Read the model definition and answer for the solid it produces. Units are mm, in the model's axes. A direction names the side the tool comes from. Coordinates: 2 decimals unless noted, no trailing zeros. Loops run counter-clockwise (first coordinate to the right, second up) from the corner with the lowest first, then second, coordinate; pieces in that order, holes last. Notation, with made-up numbers: (47.5, 69) -> (56.5, 69) arc R19 cw to (56.5, 100) -> close; hole circle Ø1 at (-15.5, -22.5). An arc over 180 degrees is marked (long way). Answer as a JSON object with one key per item and string values. Group by question number.
1) Determine the mould class of faces 5 (the face through (3, -20, -24.284)), 6 (the face through (0, -20, -14)), 7 (the face through (2, -7, -7)) for opening direction Y: released by +Y, released by -Y, zero draft, split by the parting line, or undercut.
2) Section D-D, the plane y = -23 is taken. Give the vertices of the cut face in (x, z).
3) A flat-ended cylindrical pin translates along its axis: P1, Ø1.5, axis at x = 2.5, z = -9, coming from the +Y side. Find the tip coordinate at first contact, or state that the pin passes through.
4) Section B-B, the plane x = 4.1 is taken. Give the vertices of the cut face in (y, z).
5) Consider probe 1 along Z at (x, y) = (4.1, -18.5); probe 2 along Z at (x, y) = (3.55, -30); probe 3 along Z at (x, y) = (0.35, -23). Determine where each line is inside the solid, lowest interval first. Write a range as [from, to].
6) Section C-C, the plane z = -7.75 is taken. Give the vertices of the cut face in (x, y), plus the area to 3 significant figures.
7) Which of the six approach directions +Z, -Z, +X, -X, +Y, -Y give full straight-line access (tool end or side, diameter ignored) to faces 1 (the face through (2.465, -6.972, -21.312)), 2 (the face through (2, -20, 0)), 3 (the face through (2.535, -26.329, -8.014)), 4 (the face through (2, -33, -7))?
8) Section A-A, the plane y = -3.5 is taken. Give the vertices of the cut face in (x, z), plus the area to 3 significant figures.
from build123d import *

# Parameters (mm, degrees)
BOSS_EXTRUDE1_DEPTH = 5
CUT_EXTRUDE1_DEPTH  = 50.244289009


with BuildPart() as part:
    # Sketch1 → Boss-Extrude1 (new body)
    with BuildSketch(Plane(origin=(0, 0, 0), x_dir=(0, 0, -1), z_dir=(1, 0, 0))):
        Polygon((0, 0), (0, -40), (14.142135624, -25.857864376), (28.284271247, -40), (28.284271247, 0), (14.142135624, -14.142135624), align=None)
    extrude(amount=BOSS_EXTRUDE1_DEPTH)

    # Sketch2 → Cut-Extrude1 (cut, through all)
    with BuildSketch(Plane(origin=(5, 0, 0), x_dir=(0, 0, -1), z_dir=(1, 0, 0))):
        Polygon((4, -30.343145751), (12.142135624, -22.201010127), (12.142135624, -17.798989873), (4, -9.656854249), align=None)
        Polygon((16.142135624, -17.798989873), (16.142135624, -22.201010127), (24.284271247, -30.343145751), (24.284271247, -9.656854249), align=None)
    extrude(amount=-CUT_EXTRUDE1_DEPTH, mode=Mode.SUBTRACT)


solid = part.part
Determined:
{
 "1": {"face 5": "undercut", "face 6": "zero draft", "face 7": "released by +Y"},
 "2": {"outline": "(0, -28.28) -> (5, -28.28) -> (5, -24.28) -> (0, -24.28) -> close; (0, -16.94) -> (5, -16.94) -> (5, -11.34) -> (0, -11.34) -> close; (0, -4) -> (5, -4) -> (5, 0) -> (0, 0) -> close"},
 "3": {"P1": "y = -8.25"},
 "4": {"outline": "(-40, -28.28) -> (0, -28.28) -> (-14.14, -14.14) -> (0, 0) -> (-40, 0) -> (-25.86, -14.14) -> close; hole (-30.34, -24.28) -> (-9.66, -24.28) -> (-17.8, -16.14) -> (-22.2, -16.14) -> close; hole (-30.34, -4) -> (-22.2, -12.14) -> (-17.8, -12.14) -> (-9.66, -4) -> close"},
 "5": {"probe 1": "[-28.28, -24.28], [-16.14, -12.14], [-4, 0]", "probe 2": "[-28.28, -24.28], [-23.94, -18.28], [-10, -4.34], [-4, 0]", "probe 3": "[-28.28, -24.28], [-16.94, -11.34], [-4, 0]"},
 "6": {"outline": "(0, -32.25) -> (5, -32.25) -> (5, -26.59) -> (0, -26.59) -> close; (0, -13.41) -> (5, -13.41) -> (5, -7.75) -> (0, -7.75) -> close", "area": "56.6 mm²"},
 "7": {"face 1": "+X, -X, +Y", "face 2": "+Z, +X, -X, +Y, -Y", "face 3": "+X, -X", "face 4": "+X, -X, -Y"},
 "8": {"outline": "(0, -28.28) -> (5, -28.28) -> (5, -24.78) -> (0, -24.78) -> close; (0, -3.5) -> (5, -3.5) -> (5, 0) -> (0, 0) -> close", "area": "35.0 mm²"}
}
